Check sheet for the drawn part. Datum: minimum x, y, z corner. Units: mm. Give positions to 0.01 mm unless a question says otherwise; leave off trailing zeros. Write each loop counter-clockwise with the first axis right and the second up, starting at its lowest first coordinate (ties: lowest second). Pieces come first, ordered by that corner, then holes. Notation, with made-up numbers: (68, 3) - (114, 3) arc R8 ccw to (114, 12) - close; hole circle Ø11 at (-31.75, 55.5). An arc over 180 degrees is marked (long way). Answer as a JSON object with one key per item and string values. Group by question number.
Item 1: Go/stop test with flat-tipped pins: pin 1 (1.9 mm diameter, centred on x = 50, y = 48, fed in from -Z); pin 2 (1.5 mm diameter, centred on x = 22, z = 1, fed in from -Y). Record where each tip stops, or that it passes through.
Item 2: Sectioned sample at A-A, the plane y = 18. Record the boundary of the cut face in (x, z).
Item 3: Sectioned sample at B-B, the plane x = 50. Record the boundary of the cut face in (y, z).
Item 4: Sectioned sample at C-C, the plane y = 30. Record the boundary of the cut face in (x, z), and give its area (3 significant figures).
Item 5: Scan lines: line 1 along Y through (x, z) = (50, 0.8); line 2 along Y through (x, z) = (10, 2.3); line 3 along X through (y, z) = (35.5, 0.4). Record each from-to range of solid material in increasing order. Write a range as [from, to].
Item 6: Sectioned sample at D-D, the plane z = 0.55. Record the boundary of the cut face in (x, y).
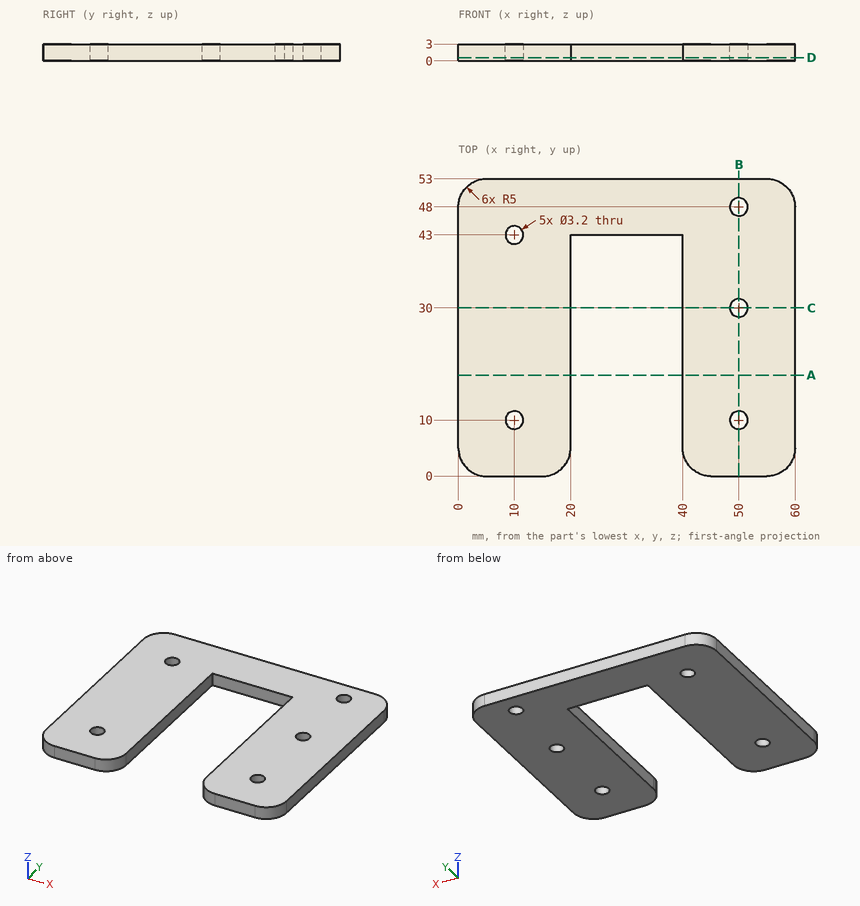
Geometry check:
{
 "1": {"pin 1": "through", "pin 2": "y = 43"},
 "2": {"outline": "(0, 0) - (20, 0) - (20, 3) - (0, 3) - close; (40, 0) - (60, 0) - (60, 3) - (40, 3) - close"},
 "3": {"outline": "(0, 0) - (8.4, 0) - (8.4, 3) - (0, 3) - close; (11.6, 0) - (28.4, 0) - (28.4, 3) - (11.6, 3) - close; (31.6, 0) - (46.4, 0) - (46.4, 3) - (31.6, 3) - close; (49.6, 0) - (53, 0) - (53, 3) - (49.6, 3) - close"},
 "4": {"outline": "(0, 0) - (20, 0) - (20, 3) - (0, 3) - close; (40, 0) - (48.4, 0) - (48.4, 3) - (40, 3) - close; (51.6, 0) - (60, 0) - (60, 3) - (51.6, 3) - close", "area": "110 mm^2"},
 "5": {"line 1": "[0, 8.4], [11.6, 28.4], [31.6, 46.4], [49.6, 53]", "line 2": "[0, 8.4], [11.6, 41.4], [44.6, 53]", "line 3": "[0, 20], [40, 60]"},
 "6": {"outline": "(0, 5) arc R5 ccw to (5, 0) - (15, 0) arc R5 ccw to (20, 5) - (20, 43) - (40, 43) - (40, 5) arc R5 ccw to (45, 0) - (55, 0) arc R5 ccw to (60, 5) - (60, 48) arc R5 ccw to (55, 53) - (5, 53) arc R5 ccw to (0, 48) - close; hole circle Ø3.2 at (10, 10); hole circle Ø3.2 at (10, 43); hole circle Ø3.2 at (50, 10); hole circle Ø3.2 at (50, 30); hole circle Ø3.2 at (50, 48)"}
}
